Input: dimensioned drawing with shaded views. Units: mm. Origin: part minimum x, y, z. Round coordinates to 2 decimals unless told otherwise and drop trailing zeros. Loops run counter-clockwise (first coordinate to the right, second up) from the corner with the lowest first, then second, coordinate; pieces in that order, holes last.
Item 1: Section query C-C on y = 2.45. Return loops of the section in (x, z).
Item 2: Ray query, L1, parallel to X at y = 1.1, z = 20; L2, parallel to X at y = 0.85, z = 117.5. Return the intervals inside material, ascending.
Item 3: Section query A-A on z = 70. Return loops of the section in (x, y).
Item 4: Section query D-D on x = 58. Return loops of the section in (y, z), then the cut area to 3 significant figures.
Item 5: Section query B-B on x = 120. Return loops of the section in (y, z), then the cut area to 3 significant figures.
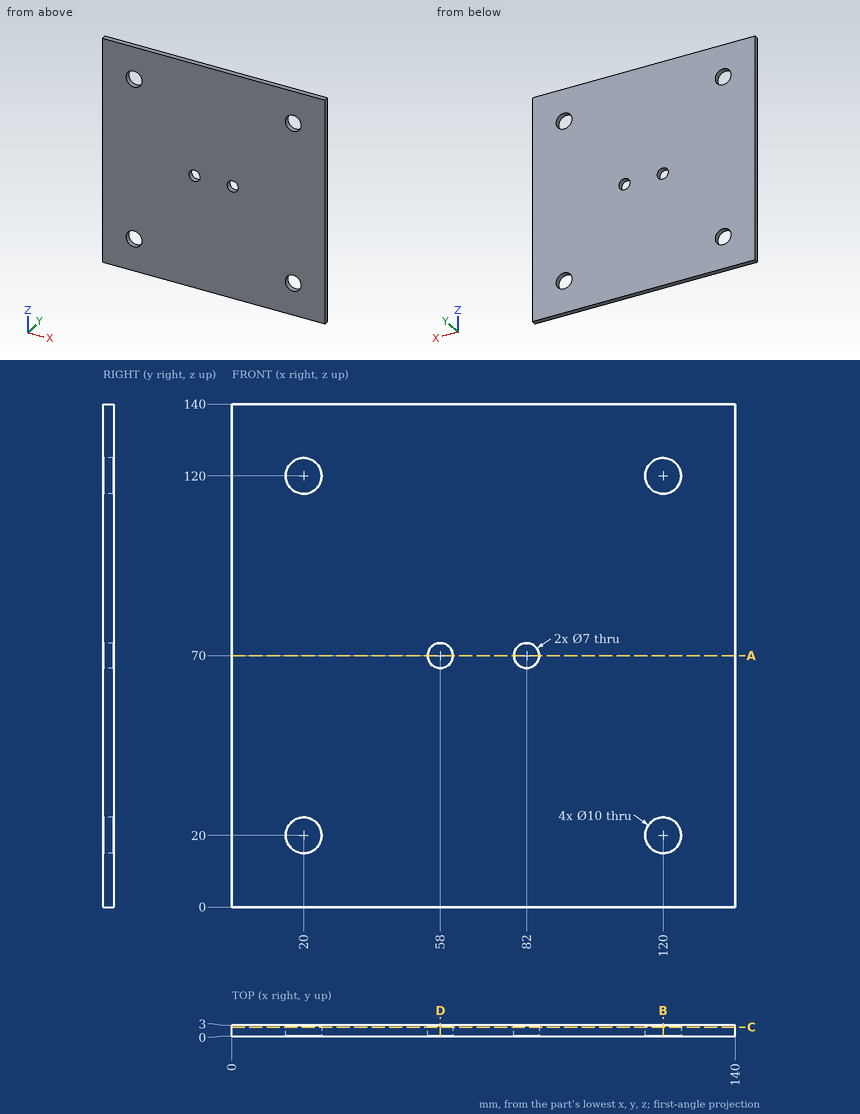
Data:
1. outline: (0, 0) - (140, 0) - (140, 140) - (0, 140) - close; hole circle Ø10 at (20, 20); hole circle Ø10 at (20, 120); hole circle Ø7 at (58, 70); hole circle Ø7 at (82, 70); hole circle Ø10 at (120, 20); hole circle Ø10 at (120, 120)
2. L1: x = 0 to 15, 25 to 115, 125 to 140
2. L2: x = 0 to 15.67, 24.33 to 115.67, 124.33 to 140
3. outline: (0, 0) - (54.5, 0) - (54.5, 3) - (0, 3) - close; (61.5, 0) - (78.5, 0) - (78.5, 3) - (61.5, 3) - close; (85.5, 0) - (140, 0) - (140, 3) - (85.5, 3) - close
4. outline: (0, 0) - (3, 0) - (3, 66.5) - (0, 66.5) - close; (0, 73.5) - (3, 73.5) - (3, 140) - (0, 140) - close
4. area: 399 mm2
5. outline: (0, 0) - (3, 0) - (3, 15) - (0, 15) - close; (0, 25) - (3, 25) - (3, 115) - (0, 115) - close; (0, 125) - (3, 125) - (3, 140) - (0, 140) - close
5. area: 360 mm2
